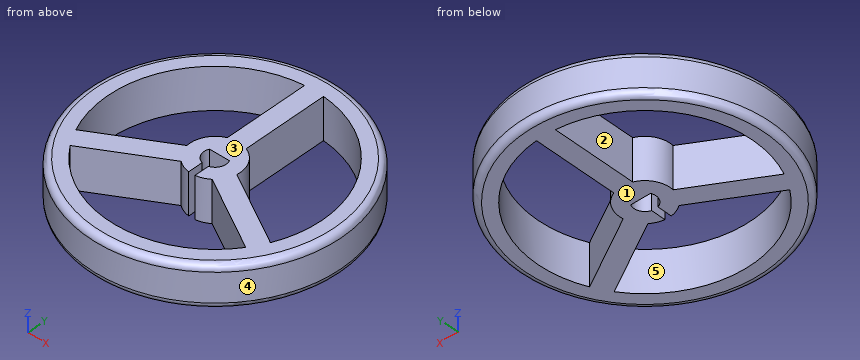
Autodesk Inventor part; units mm, degrees
ref_plane "YZ Plane" through (0, 0, 0) normal (1, 0, 0) x (0, 1, 0)
ref_plane "XZ Plane" through (0, 0, 0) normal (0, 1, 0) x (-1, 0, 0)
ref_plane "XY Plane" through (0, 0, 0) normal (0, 0, 1) x (1, 0, 0)
sketch "Sketch1" plane through (0, 0, 0) normal (0, 0, 1) x (1, 0, 0)
  circle A0 centre (0, 0) radius 20
  dimension "d0" = 40
extrude "Extrusion1" add sketch "Sketch1" along normal blind 6.6
sketch "Sketch3" plane through (0, 0, 0) normal (0, 0, -1) x (-1, 0, 0)
  circle A0 centre (0, 0) radius 17
  line L0 (0, 17) -> (0, 0)
  line L1 (0, 0) -> (14.7224, -8.5)
  line L2 (0, 0) -> (-14.7224, -8.5)
  line L3 (0, 0) -> (17, 0) construction
  line L4 (1.5, 16.9337) -> (1.5, 0.866)
  line L5 (-1.5, 16.9337) -> (-1.5, 0.866)
  line L6 (-1.5, 0.866) -> (-15.415, -7.1678)
  line L7 (0, -1.7321) -> (-13.915, -9.7659)
  line L8 (1.5, 0.866) -> (15.415, -7.1678)
  line L9 (0, -1.7321) -> (13.915, -9.7659)
  dimension "d6" = 34
  dimension "d7" = 120
  dimension "d8" = 150
  dimension "d9" = 1.5
  dimension "d10" = 1.5
  dimension "d11" = 1.5
  dimension "d12" = 1.5
  dimension "d13" = 1.5
  dimension "d14" = 1.5
extrude "Extrusion3" cut sketch "Sketch3" against normal up to surface (6.6 mm away) contours A0 L8 L4 | L5 L6 A0 | A0 L7 L9
sketch "Sketch5" plane through (0, 0, 6.6) normal (0, 0, 1) x (1, 0, 0)
  circle A0 centre (0, 0) radius 4
  dimension "d20" = 8
extrude "Extrusion5" add sketch "Sketch5" against normal blind 6.6
sketch "Sketch6" plane through (0, 0, 0) normal (0, 0, -1) x (-1, 0, 0)
  circle A0 centre (0, 0) radius 1.75
  line L0 (0, -1.75) -> (0, -4)
  arc A1 (-2.4613, -3.1531) -> (2.4613, -3.1531) centre (0, 0) ccw
  line L1 (0.5, -1.6771) -> (0.5, -3.9686)
  line L2 (-0.5, -1.6771) -> (-0.5, -3.9686)
  line L3 (-1.5811, 0.75) -> (1.5811, 0.75)
  point P0 (0.0845, 0.75)
  dimension "d23" = 3.5
  dimension "d24" = 0.5
  dimension "d25" = 0.5
  dimension "d29" = 2.5
extrude "Extrusion6" cut sketch "Sketch6" against normal up to surface (6.6 mm away) contours A0 L3 | L1 A1 L0 A0 | L0 A1 L2 A0 picked at (0, -0.0833)
fillet "Arredondamento1" radius 1 2 edges at (-20, 0, 6.6) (-20, 0, 0)
properties part number "wheel"
Model file for the job. Use its own axes, mm. Face numbers are marked on the shaded views. A direction names the side the tool comes from. Give positions to 0.01 mm unless a question says otherwise; leave off trailing zeros. Loops run counter-clockwise (first coordinate to the right, second up) from the corner with the lowest first, then second, coordinate; pieces in that order, holes last. Notation, with made-up numbers: M 17.25,58.25 L 63.25,58.25 A21 ccw 63.25,62.25 Z; hole C 11,75 d7. An arc over 180 degrees is marked long. Use one line per item in the form item = value.
Item 1: Slice it at A-A on y = 0. List the corners of the cut face in (x, z), and give its area (3 significant figures).
Filled in:
outline = M -20,1 A1 ccw -19,0 L -17,0 L -17,6.6 L -19,6.6 A1 ccw -20,5.6 Z; M -4,0 L -1.75,0 L -1.75,6.6 L -4,6.6 Z; M 1.75,0 L 4,0 L 4,6.6 L 1.75,6.6 Z; M 17,0 L 19,0 A1 ccw 20,1 L 20,5.6 A1 ccw 19,6.6 L 17,6.6 Z
area = 68.4 mm^2
Item 2: Slice it at B-B on x = 0. List the corners of the cut face in (y, z), and give its area (3 significant figures).
Filled in:
outline = M -20,1 A1 ccw -19,0 L -17,0 L -17,6.6 L -19,6.6 A1 ccw -20,5.6 Z; M 0.75,0 L 19,0 A1 ccw 20,1 L 20,5.6 A1 ccw 19,6.6 L 0.75,6.6 Z
area = 146 mm^2
Item 3: Which spindle directions (+Z, -Z, +X, -X, +Y, -Y) get a long thin tool onto all of the face, cutting with end or side? Do the marked faces 1 and 2. Say none if no direction does.
Filled in:
face_1 = -Z, +X, -X, +Y, -Y
face_2 = +Z, -Z
Item 4: Two-plate mould, pull along X, no slides. Class the marked faces 3, 4 and 5: released by +X, released by -X, zero draft, split by the parting line, or undercut.
Filled in:
face_3 = zero draft
face_4 = split by the parting line
face_5 = undercut
Item 5: Drill centre lines: L1, parallel to Y at x = 11, z = 0.75; L2, parallel to Y at x = 3.5, z = 2.25; L3, parallel to X at y = 9, z = 3.25. Where is each one in solid material? Low to high.
Filled in:
L1 = -16.67 to -12.96, -8.08 to -4.62, 12.96 to 16.67
L2 = -19.69 to -16.64, -3.75 to 1.94, 16.64 to 19.69
L3 = -17.86 to -14.42, -1.5 to 1.5, 14.42 to 17.86
Item 6: Slice it at D-D on y = 13. Give the number of separate pieces and of enclosed holes in the cut face, and give its area (3 significant figures).
Filled in:
separate_pieces = 3
enclosed_holes = 0
area = 74.7 mm^2
Item 7: Slice it at C-C on z = 3.25. List the corners of the cut face in (x, y) (3 decimals), and give its area (3 significant figures).
Filled in:
outline = C 0,0 d40; hole M -15.415,-7.168 L -3.961,-0.555 A4 cw -1.5,3.708 L -1.5,16.934 A17 ccw Z; hole M -13.915,-9.766 A17 ccw 13.915,-9.766 L 2.461,-3.153 A4 cw 0.5,-3.969 L 0.5,-1.677 A1.75 ccw 1.581,0.75 L -1.581,0.75 A1.75 ccw -0.5,-1.677 L -0.5,-3.969 A4 cw -2.461,-3.153 Z; hole M 1.5,3.708 A4 cw 3.961,-0.555 L 15.415,-7.168 A17 ccw 1.5,16.934 Z
area = 507 mm^2
Item 8: Flat gauge pins, fed straight in: pin 1 Ø3.5 at (y, z) = (8, 2) entering from +X; pin 2 Ø2 at (x, z) = (14, 5) entering from -Y; pin 3 Ø2.5 at (y, z) = (-3, 2) entering from -X; pin 4 Ø2 at (x, y) = (8, -12) entering from +Z. Where does each tip first touch, or does it go through?
Filled in:
pin_1 = 19
pin_2 = -15.2
pin_3 = -19.92
pin_4 = through
